```python
from build123d import *

# Parameters (mm, degrees)
SKETCH1_W           = 47
SKETCH1_H           = 35
BOSS_EXTRUDE1_DEPTH = 8.5
SKETCH2_W           = 4.3
SKETCH2_H           = 1.5
SKETCH2_W_2         = 1.5
SKETCH2_H_2         = 4.3
BOSS_EXTRUDE2_DEPTH = 5
SKETCH3_W           = 4.3
SKETCH3_H           = 1.5
SKETCH3_W_2         = 1.5
SKETCH3_H_2         = 4.3
CUT_EXTRUDE1_DEPTH  = 5


with BuildPart() as part:
    # Sketch1 → Boss-Extrude1 (new body)
    with BuildSketch(Plane(origin=(0, 0, 0), x_dir=(1, 0, 0), z_dir=(0, 1, 0))):
        Rectangle(SKETCH1_W, SKETCH1_H)
    extrude(amount=BOSS_EXTRUDE1_DEPTH)

    # Sketch2 → Boss-Extrude2 (add)
    with BuildSketch(Plane(origin=(0, 0, 0), x_dir=(-1, 0, 0), z_dir=(0, -1, 0))):
        with Locations((0, 18.25)):
            Rectangle(SKETCH2_W, SKETCH2_H)
        with Locations((-24.25, 0)):
            Rectangle(SKETCH2_W_2, SKETCH2_H_2)
    extrude(amount=-BOSS_EXTRUDE2_DEPTH)

    # Sketch3 → Cut-Extrude1 (cut)
    with BuildSketch(Plane(origin=(0, 0, 0), x_dir=(-1, 0, 0), z_dir=(0, -1, 0))):
        with Locations((0, -16.75)):
            Rectangle(SKETCH3_W, SKETCH3_H)
        with Locations((22.75, 0)):
            Rectangle(SKETCH3_W_2, SKETCH3_H_2)
    extrude(amount=-CUT_EXTRUDE1_DEPTH, mode=Mode.SUBTRACT)


solid = part.part
```
Can you work these out from the model? Positions are in its coordinate system, mm. A direction names the side the tool comes from. Round coordinates to 2 decimals unless told otherwise and drop trailing zeros. Loops run counter-clockwise (first coordinate to the right, second up) from the corner with the lowest first, then second, coordinate; pieces in that order, holes last. Notation, with made-up numbers: M -17,4.5 L 20,4.5 A12 ccw 20,23.5 Z; hole C -28.75,40 d10. An arc over 180 degrees is marked long. Answer as a JSON object with one key per item and string values. Group by question number.
Q1. Imagine slicing it at C-C, the plane z = 14.5. Please give me the cut outline in (x, y).
Q2. Imagine slicing it at A-A, the plane x = -1. Please give me the cut outline in (y, z).
Q3. Please list where these lines run through material, in increasing order: L1, parallel to X at y = 7.75, z = -10; L2, parallel to Z at x = 21.5, y = 5.75; L3, parallel to X at y = 4, z = 1.
Q4. Imagine slicing it at B-B, the plane y = 7.5. Please give me the cut outline in (x, z), then the cut area to 4 significant figures.
Q5. On a 3-axis mill with a long thin cutter (end or side, diameter ignored), from which of +Z, -Z, +X, -X, +Y, -Y can I reach the whole of each face in a straight line? I mean faces 1 (the flat face through (24, 2, 2.15)), 2 (the flat face through (-23, 2, -2.15)), 3 (the flat face through (0, 5, 17)), 4 (the flat face through (-2.15, 2, -18)), 5 (the flat face through (24, 5, 0)). Say none if no direction works.
Q6. We'd pull the mould along Z, two halves only. Please class faces 6 (the flat face through (24, 2, -2.15)), 7 (the flat face through (-23, 5, 0)), 8 (the flat face through (2.15, 2, -18)), 9 (the flat face through (0, 6, 17.5)): +Z half, -Z half, draft (parallel to the pull), parting line (faces both ways), or undercut.
Q7. Will these pins go through, and if not, where does the flat tip stop? pin 1 (8 mm diameter, centred on x = -2.5, z = -14, fed in from -Y); pin 2 (2.5 mm diameter, centred on y = 6, z = -8.5, fed in from +X); pin 3 (0.8 mm diameter, centred on y = 3, z = -18, fed in from -X); pin 4 (2 mm diameter, centred on x = -10, y = 3.5, fed in from -Z).
Findings:
{
 "1": {"outline": "M -23.5,0 L 23.5,0 L 23.5,8.5 L -23.5,8.5 Z"},
 "2": {"outline": "M 0,-19 L 5,-19 L 5,-17.5 L 8.5,-17.5 L 8.5,17.5 L 5,17.5 L 5,16 L 0,16 Z"},
 "3": {"L1": "x = -23.5 to 23.5", "L2": "z = -17.5 to 17.5", "L3": "x = -22 to 25"},
 "4": {"outline": "M -23.5,-17.5 L 23.5,-17.5 L 23.5,17.5 L -23.5,17.5 Z", "area": "1,645 mm2"},
 "5": {"face 1": "+Z, +X, +Y, -Y", "face 2": "-X, -Y", "face 3": "+Z, -Y", "face 4": "-Z, -X, +Y, -Y", "face 5": "+Z, -Z, +X, +Y"},
 "6": {"face 6": "-Z half", "face 7": "undercut", "face 8": "draft", "face 9": "+Z half"},
 "7": {"pin 1": "stops at y = 0", "pin 2": "stops at x = 23.5", "pin 3": "stops at x = -2.15", "pin 4": "stops at z = -17.5"}
}
